Check sheet for the modelled part. Datum: model origin and axes. Units: mm. Face numbers are marked on the shaded views. A direction names the side the tool comes from. Give positions to 0.01 mm unless a question says otherwise; leave off trailing zeros. Write each loop counter-clockwise with the first axis right and the second up, starting at its lowest first coordinate (ties: lowest second). Pieces come first, ordered by that corner, then holes. Notation, with made-up numbers: (8, -32) -> (40, -32) arc R15 cw to (40, -15) -> close; hole circle Ø9 at (86.25, -27). An arc over 180 degrees is marked (long way). Return JSON: item names as keys, results as strings.
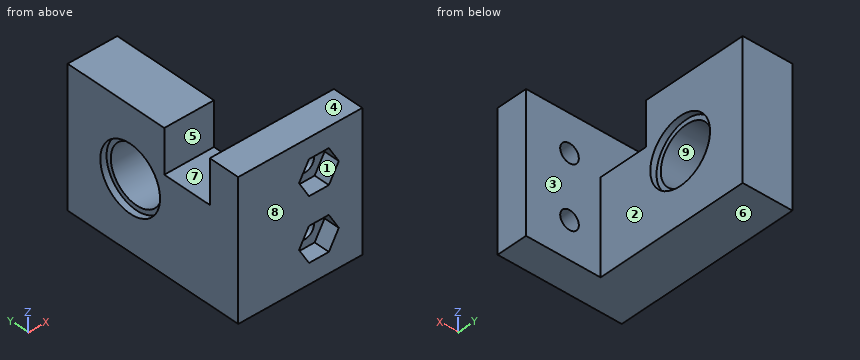
from build123d import *

# Parameters (mm, degrees)
SKETCH_1_W               = 40
SKETCH_1_H               = 23
SKETCH_1_R               = 4.5
EXTRUDE_1_DEPTH          = 8
SKETCH_2_R               = 5.25
CUT_EXTRUDE_1_DEPTH      = 1
CUT_EXTRUDE_2_DEPTH      = 9
SKETCH_5_R               = 5.25
CUT_EXTRUDE_3_DEPTH      = 1
SKETCH_6_W               = 22
SKETCH_6_H               = 5
EXTRUDE_3_DEPTH          = 6
SKETCH_7_W               = 11
SKETCH_7_H               = 4
EXTRUDE_4_DEPTH          = 4
EXTRUDE_6_DEPTH          = 3
SKETCH_12_W              = 8
SKETCH_12_H              = 15
EXTRUDE_7_DEPTH          = 13
SKETCH_13_W              = 22
SKETCH_13_H              = 5
EXTRUDE_8_DEPTH          = 10
SKETCH_14_W              = 6
SKETCH_14_H              = 22
CUT_EXTRUDE_9_DEPTH      = 13
CUT_EXTRUDE_9_DEPTH_BACK = 10
SKETCH_15_R              = 1.5
CUT_EXTRUDE_10_DEPTH     = 6
CUT_EXTRUDE_11_DEPTH     = 2.5
SKETCH_17_W              = 22
SKETCH_17_H              = 5
EXTRUDE_9_DEPTH          = 2
SKETCH_18_W              = 8
SKETCH_18_H              = 5
EXTRUDE_10_DEPTH         = 7


with BuildPart() as part:
    # 草图1 → 凸台-拉伸1 (new body)
    with BuildSketch(Plane(origin=(0, 0, 0), x_dir=(0, 0, -1), z_dir=(1, 0, 0))):
        with Locations((9, 5.5)):
            Rectangle(SKETCH_1_W, SKETCH_1_H)
        Circle(SKETCH_1_R, mode=Mode.SUBTRACT)
        with Locations((18, 6)):
            Circle(SKETCH_1_R, mode=Mode.SUBTRACT)
    extrude(amount=EXTRUDE_1_DEPTH)

    # 草图2 → 切除-拉伸1 (cut)
    with BuildSketch(Plane.ZY):
        with Locations((-18, 6)):
            Circle(SKETCH_2_R)
        Circle(SKETCH_2_R)
    extrude(amount=-CUT_EXTRUDE_1_DEPTH, mode=Mode.SUBTRACT)

    # 草图3 → 切除-拉伸2 (cut, through all)
    with BuildSketch(Plane(origin=(8, 0, 0), x_dir=(0, 0, -1), z_dir=(1, 0, 0))):
        Polygon((29, 17), (11, 17), (-11, 17), (-11, 11), (11, 11), (11, -6), (29, -6), align=None)
    extrude(amount=-CUT_EXTRUDE_2_DEPTH, mode=Mode.SUBTRACT)

    # 草图5 → 切除-拉伸3 (cut)
    with BuildSketch(Plane(origin=(8, 0, 0), x_dir=(0, 0, -1), z_dir=(1, 0, 0))):
        Circle(SKETCH_5_R)
    extrude(amount=-CUT_EXTRUDE_3_DEPTH, mode=Mode.SUBTRACT)

    # 草图6 → 凸台-拉伸3 (add)
    with BuildSketch(Plane(origin=(8, 0, 0), x_dir=(0, 0, -1), z_dir=(1, 0, 0))):
        with Locations((0, -3.5)):
            Rectangle(SKETCH_6_W, SKETCH_6_H)
    extrude(amount=EXTRUDE_3_DEPTH)

    # 草图7 → 凸台-拉伸4 (add)
    with BuildSketch(Plane.XZ.offset(6)):
        with Locations((8.5, -9)):
            Rectangle(SKETCH_7_W, SKETCH_7_H)
    extrude(amount=EXTRUDE_4_DEPTH)

    # 草图11 → 凸台-拉伸6 (add)
    with BuildSketch(Plane(origin=(0, 0, -11), x_dir=(-1, 0, 0), z_dir=(0, 0, -1))):
        Polygon((-8, -1), (-8, 11), (-14, -1), align=None)
    extrude(amount=-EXTRUDE_6_DEPTH)

    # 草图12 → 凸台-拉伸7 (add)
    with BuildSketch(Plane.XZ.offset(6)):
        with Locations((4, -3.5)):
            Rectangle(SKETCH_12_W, SKETCH_12_H)
    extrude(amount=EXTRUDE_7_DEPTH)

    # 草图13 → 凸台-拉伸8 (add)
    with BuildSketch(Plane(origin=(8, 0, 0), x_dir=(0, 0, -1), z_dir=(1, 0, 0))):
        with Locations((0, -16.5)):
            Rectangle(SKETCH_13_W, SKETCH_13_H)
    extrude(amount=EXTRUDE_8_DEPTH)

    # 草图14 → 切除-拉伸9 (cut, two sides)
    with BuildSketch(Plane(origin=(0, -1, 0), x_dir=(1, 0, 0), z_dir=(0, 1, 0))) as cut_extrude_9_sk:
        with Locations((11, 0)):
            Rectangle(SKETCH_14_W, SKETCH_14_H)
    extrude(amount=CUT_EXTRUDE_9_DEPTH, mode=Mode.SUBTRACT)
    extrude(cut_extrude_9_sk.sketch, amount=-CUT_EXTRUDE_9_DEPTH_BACK, mode=Mode.SUBTRACT)

    # 草图15 → 切除-拉伸10 (cut, through all)
    with BuildSketch(Plane(origin=(0, -14, 0), x_dir=(-1, 0, 0), z_dir=(0, 1, 0))):
        with Locations((-13, -5)):
            Circle(SKETCH_15_R)
        with Locations((-13, 5)):
            Circle(SKETCH_15_R)
    extrude(amount=-CUT_EXTRUDE_10_DEPTH, mode=Mode.SUBTRACT)

    # 草图16 → 切除-拉伸11 (cut)
    with BuildSketch(Plane.XZ.offset(19)):
        Polygon((16.204293994, 5), (14.602146997, 7.775), (11.397853003, 7.775), (9.795706006, 5), (11.397853003, 2.225), (14.602146997, 2.225), align=None)
        Polygon((16.204293994, -5), (14.602146997, -2.225), (11.397853003, -2.225), (9.795706006, -5), (11.397853003, -7.775), (14.602146997, -7.775), align=None)
    extrude(amount=-CUT_EXTRUDE_11_DEPTH, mode=Mode.SUBTRACT)

    # 草图17 → 凸台-拉伸9 (add)
    with BuildSketch(Plane(origin=(18, 0, 0), x_dir=(0, 0, -1), z_dir=(1, 0, 0))):
        with Locations((0, -16.5)):
            Rectangle(SKETCH_17_W, SKETCH_17_H)
    extrude(amount=EXTRUDE_9_DEPTH)

    # 草图18 → 凸台-拉伸10 (add, through all)
    with BuildSketch(Plane.XY.offset(4)):
        with Locations((4, -16.5)):
            Rectangle(SKETCH_18_W, SKETCH_18_H)
    extrude(amount=EXTRUDE_10_DEPTH)


solid = part.part
(1) Depth check by flat-ended pin: pin 1 Ø12 at (y, z) = (0, 0) entering from -X; pin 2 Ø11.5 at (y, z) = (0, 0) entering from +X; pin 3 Ø3 at (x, z) = (13.5, 4.5) entering from -Y; pin 4 Ø5 at (y, z) = (0.5, 2) entering from +X. Enter the tip coordinate at first touch or a pass-through.
Reply:
{"pin 1": "x = 0", "pin 2": "x = 8", "pin 3": "y = -16.5", "pin 4": "x = 7"}
(2) Set-up check for the marked faces 1, 2, 3, 4 and 5: record each of +Z, -Z, +X, -X, +Y, -Y from which the full face is reachable in a straight line by a thin tool's end or side.
Reply:
{"face 1": "-Y", "face 2": "+Z, -Z, +X, +Y", "face 3": "+Z, +X", "face 4": "+Z, +X, -X, +Y, -Y", "face 5": "+Z, +X, -X"}
(3) Thickness scan on L1, parallel to Z at x = 13, y = -15.3; L2, parallel to Y at x = 3.9, z = 0; L3, parallel to Z at x = 7.7, y = 0. Record the ranges inside material, lowest first.
Reply:
{"L1": "-11 to -6.5, -3.5 to 3.5, 6.5 to 11", "L2": "-19 to -4.5, 4.5 to 11", "L3": "-11 to -5.25, 5.25 to 11"}
(4) Cross-section at C-C on x = 6. Enter the section's corners in (y, z).
Reply:
{"outline": "(-19, -11) -> (11, -11) -> (11, 11) -> (-6, 11) -> (-6, 4) -> (-14, 4) -> (-14, 11) -> (-19, 11) -> close; hole circle Ø9 at (0, 0)"}
(5) Cross-section at B-B on y = 0. Enter the section's corners in (x, z), then the cut area to 3 significant figures.
Reply:
{"outline": "(0, -11) -> (8, -11) -> (8, -5.25) -> (7, -5.25) -> (7, -4.5) -> (1, -4.5) -> (1, -5.25) -> (0, -5.25) -> close; (0, 5.25) -> (1, 5.25) -> (1, 4.5) -> (7, 4.5) -> (7, 5.25) -> (8, 5.25) -> (8, 11) -> (0, 11) -> close", "area": "101 mm^2"}
(6) Cross-section at A-A on x = 13. Enter the section's corners in (y, z) (3 decimals).
Reply:
{"outline": "(-19, -11) -> (-14, -11) -> (-14, -6.5) -> (-16.5, -6.5) -> (-16.5, -7.775) -> (-19, -7.775) -> close; (-19, -2.225) -> (-16.5, -2.225) -> (-16.5, -3.5) -> (-14, -3.5) -> (-14, 3.5) -> (-16.5, 3.5) -> (-16.5, 2.225) -> (-19, 2.225) -> close; (-19, 7.775) -> (-16.5, 7.775) -> (-16.5, 6.5) -> (-14, 6.5) -> (-14, 11) -> (-19, 11) -> close"}
(7) Release check for a two-part mould opening along Y. For the marked faces 6, 7, 8 and 9 record: pulls with the +Y half, pulls with the -Y half, needs draft (parallel to the pull), parting line crosses it, or undercut.
Reply:
{"face 6": "needs draft", "face 7": "undercut", "face 8": "pulls with the -Y half", "face 9": "undercut"}
(8) Cross-section at D-D on z = -1. Enter the section's corners in (x, y).
Reply:
{"outline": "(0, -19) -> (20, -19) -> (20, -14) -> (8, -14) -> (8, -5.15) -> (7, -5.15) -> (7, -4.39) -> (1, -4.39) -> (1, -5.15) -> (0, -5.15) -> close; (0, 5.15) -> (1, 5.15) -> (1, 4.39) -> (7, 4.39) -> (7, 5.15) -> (8, 5.15) -> (8, 11) -> (0, 11) -> close"}
